CAD build for the part. Positions are in the model's coordinates, mm. A direction names the side the tool comes from. Round coordinates to 2 decimals unless told otherwise and drop trailing zeros. Write each loop counter-clockwise with the first axis right and the second up, starting at its lowest first coordinate (ties: lowest second). Pieces come first, ordered by that corner, then holes. Notation, with made-up numbers: M 84,-24.5 L 140,-24.5 A29 ccw 140,4.5 Z; hole C 76,85.5 d5. An arc over 180 degrees is marked long. Write each question's results on one line, items separated by ' | '. Start each with the question number.
```python
from build123d import *

# Parameters (mm, degrees)
SKETCH1_W               = 15
SKETCH1_H               = 10
BOSS_EXTRUDE1_DEPTH     = 1.6
FILLET1_R               = 1.5
SKETCH2_R               = 3.45
BOSS_EXTRUDE2_DEPTH     = 1.4
SKETCH2_3_R             = 2.5
CUT_EXTRUDE1_DEPTH      = 1.4
CUT_EXTRUDE1_DEPTH_BACK = 1.6
FILLET2_R               = 1


with BuildPart() as part:
    # Sketch1 → Boss-Extrude1 (new body)
    with BuildSketch(Plane.XY):
        with Locations((7.5, 5)):
            Rectangle(SKETCH1_W, SKETCH1_H)
    extrude(amount=BOSS_EXTRUDE1_DEPTH)

    # Fillet1
    fillet1_edges = [part.edges().sort_by_distance(p)[0] for p in [
        (0, 10, 0.8),
        (15, 10, 0.8),
        (15, 0, 0.8),
        (0, 0, 0.8),
    ]]
    fillet(fillet1_edges, radius=FILLET1_R)

    # Sketch2 → Boss-Extrude2 (add)
    with BuildSketch(Plane.XY.offset(1.6)):
        with Locations((7.5, 5)):
            Circle(SKETCH2_R)
    extrude(amount=BOSS_EXTRUDE2_DEPTH)

    # Sketch2_3 → Cut-Extrude1 (cut, two sides)
    with BuildSketch(Plane.XY.offset(1.6)) as cut_extrude1_sk:
        with Locations((7.5, 5)):
            Circle(SKETCH2_3_R)
    extrude(amount=CUT_EXTRUDE1_DEPTH, mode=Mode.SUBTRACT)
    extrude(cut_extrude1_sk.sketch, amount=-CUT_EXTRUDE1_DEPTH_BACK, mode=Mode.SUBTRACT)

    # Fillet2
    fillet2_edges = [part.edges().sort_by_distance(p)[0] for p in [
        (4.05, 5, 1.6),
    ]]
    fillet(fillet2_edges, radius=FILLET2_R)


solid = part.part
```
1) Wall check: line 1 along Y through (x, z) = (7.5, 0.35); line 2 along Y through (x, z) = (7, 0.1); line 3 along Z through (x, y) = (2, 4.5). Give the ranges that are in metal, low to high. Write a range as from..to.
2) 3-axis set-ups, long thin cutter, end or side, ignore diameter. For faces 1 (the face through (0.43, 0.45, 0.81)), 2 (the face through (11, 8, 1.6)): which of +Z, -Z, +X, -X, +Y, -Y reach the whole face in a straight line?
3) Saw through at B-B, the plane x = 7.5. Write the cut outline in (y, z).
4) Saw through at D-D, the plane z = 2.3. Write the cut outline in (x, y).
5) Saw through at A-A, the plane z = 0.8. Write the cut outline in (x, y), plus the area to 3 significant figures.
6) Saw through at C-C, the plane y = 5. Write the cut outline in (x, z), plus the area to 3 significant figures.
Filled sheet:
1) line 1: y = 0..2.5, 7.5..10 | line 2: y = 0..2.55, 7.45..10 | line 3: z = 0..1.6
2) face 1: +Z, -Z, -X, -Y | face 2: +Z
3) outline: M 0,0 L 2.5,0 L 2.5,3 L 1.55,3 L 1.55,2.6 A1 cw 0.55,1.6 L 0,1.6 Z; M 7.5,0 L 10,0 L 10,1.6 L 9.45,1.6 A1 cw 8.45,2.6 L 8.45,3 L 7.5,3 Z
4) outline: C 7.5,5 d6.99; hole C 7.5,5 d5
5) outline: M 0,1.5 A1.5 ccw 1.5,0 L 13.5,0 A1.5 ccw 15,1.5 L 15,8.5 A1.5 ccw 13.5,10 L 1.5,10 A1.5 ccw 0,8.5 Z; hole C 7.5,5 d5 | area: 128 mm^2
6) outline: M 0,0 L 5,0 L 5,3 L 4.05,3 L 4.05,2.6 A1 cw 3.05,1.6 L 0,1.6 Z; M 10,0 L 15,0 L 15,1.6 L 11.95,1.6 A1 cw 10.95,2.6 L 10.95,3 L 10,3 Z | area: 19.1 mm^2
